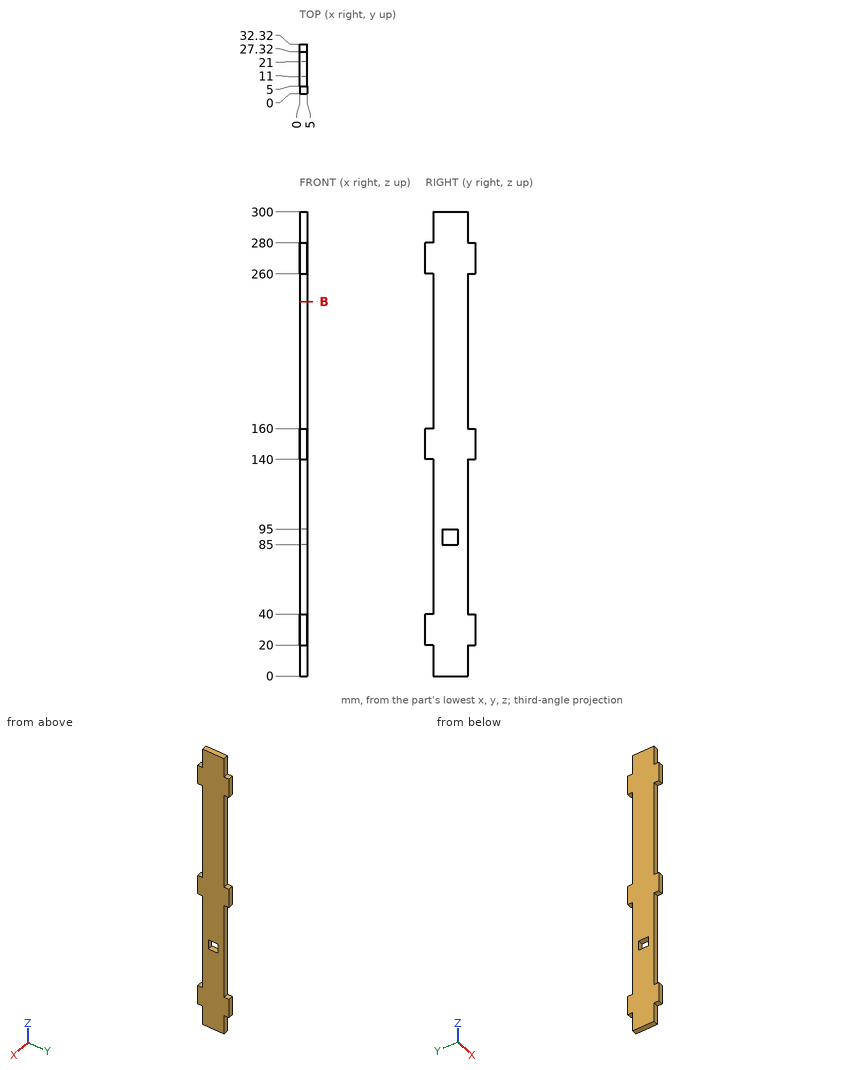
Check sheet for the drawn part. Datum: minimum x, y, z corner. Units: mm. Coordinates: 2 decimals unless noted, no trailing zeros. Order: outer loops, then holes, each group sorted by start corner. A loop starts at its lowest first (then second) coordinate and runs counter-clockwise, first axis right, second up. Notation, with made-up numbers: (6.5, 7.5) -> (17.5, 7.5) arc R19 ccw to (17.5, 11.5) -> close; hole circle Ø10 at (80, 21). An arc over 180 degrees is marked (long way). Write each question's results on one line, items separated by ' | '. Start each with the question number.
1) Material ranges on line 1 along Z through (x, y) = (2.8, 30.5); line 2 along Z through (x, y) = (3.75, 16.5); line 3 along Y through (x, z) = (1.45, 89), recorded low to high.
2) Depth check by flat-ended pin: pin 1 (2.5 mm diameter, centred on x = 2.5, y = 3.5, fed in from -Z); pin 2 (1.5 mm diameter, centred on x = 3.5, z = 111.5, fed in from -Y). Enter the tip coordinate at first touch or a pass-through.
3) Section check B-B (z = 242). Enter the section's corners in (x, y).
Checked values:
1) line 1: 20 to 40, 140 to 160, 260 to 280 | line 2: 0 to 85, 95 to 300 | line 3: 5 to 11, 21 to 27.32
2) pin 1: z = 20 | pin 2: y = 5
3) outline: (0, 5) -> (5, 5) -> (5, 27.32) -> (0, 27.32) -> close
